Can you work these out from the model? Positions are in its coordinate system, mm. A direction names the side the tool comes from. Round coordinates to 2 decimals unless told otherwise and drop trailing zeros. Loops run counter-clockwise (first coordinate to the right, second up) from the corner with the lowest first, then second, coordinate; pieces in that order, holes last. Notation, with made-up numbers: M -32.75,15 L -23.75,15 A33 ccw -23.75,50 Z; hole C -29,5.5 d6. An arc over 180 degrees is marked long. Return JSON: item names as keys, results as strings.
```python
from build123d import *

# Parameters (mm, degrees)
SKETCH1_W               = 6.3
SKETCH1_H               = 5.3
BOSS_EXTRUDE1_DEPTH     = 2
SKETCH2_W               = 0.25
SKETCH2_H               = 1.2
BOSS_EXTRUDE2_DEPTH     = 1.3
LPATTERN1_COUNT         = 8
LPATTERN1_PITCH         = 0.65
MIRROR1_COPY_1_SKETCH_W = 0.25
MIRROR1_COPY_1_SKETCH_H = 1.2
MIRROR1_COPY_1_DEPTH    = 1.3
MIRROR1_COPY_2_SKETCH_W = 0.25
MIRROR1_COPY_2_SKETCH_H = 1.2
MIRROR1_COPY_2_DEPTH    = 1.3
MIRROR1_COPY_3_SKETCH_W = 0.25
MIRROR1_COPY_3_SKETCH_H = 1.2
MIRROR1_COPY_3_DEPTH    = 1.3
MIRROR1_COPY_4_SKETCH_W = 0.25
MIRROR1_COPY_4_SKETCH_H = 1.2
MIRROR1_COPY_4_DEPTH    = 1.3
MIRROR1_COPY_5_SKETCH_W = 0.25
MIRROR1_COPY_5_SKETCH_H = 1.2
MIRROR1_COPY_5_DEPTH    = 1.3
MIRROR1_COPY_6_SKETCH_W = 0.25
MIRROR1_COPY_6_SKETCH_H = 1.2
MIRROR1_COPY_6_DEPTH    = 1.3
MIRROR1_COPY_7_SKETCH_W = 0.25
MIRROR1_COPY_7_SKETCH_H = 1.2
MIRROR1_COPY_7_DEPTH    = 1.3


with BuildPart() as part:
    # Sketch1 → Boss-Extrude1 (new body)
    with BuildSketch(Plane(origin=(0, 0, 0), x_dir=(1, 0, 0), z_dir=(0, 1, 0))):
        Rectangle(SKETCH1_W, SKETCH1_H)
    extrude(amount=BOSS_EXTRUDE1_DEPTH)

    # Sketch2 → Boss-Extrude2 (add)
    with BuildSketch(Plane.XY.offset(2.65)):
        with Locations((-2.28, 0.6)):
            Rectangle(SKETCH2_W, SKETCH2_H)
    boss_extrude2 = extrude(amount=BOSS_EXTRUDE2_DEPTH)

    # LPattern1: Boss-Extrude2 ×8
    with Locations(*[(i * LPATTERN1_PITCH, 0, 0) for i in range(1, LPATTERN1_COUNT)]):
        add(boss_extrude2)

    # Mirror1: Boss-Extrude2 across plane
    add(boss_extrude2.mirror(Plane.XY))

    # Mirror1 copy 1 sketch → Mirror1 copy 1 (add)
    with BuildSketch(Plane(origin=(0.65, 0, -2.65), x_dir=(1, 0, 0), z_dir=(0, 0, -1))):
        with Locations((-2.28, -0.6)):
            Rectangle(MIRROR1_COPY_1_SKETCH_W, MIRROR1_COPY_1_SKETCH_H)
    extrude(amount=MIRROR1_COPY_1_DEPTH)

    # Mirror1 copy 2 sketch → Mirror1 copy 2 (add)
    with BuildSketch(Plane(origin=(1.3, 0, -2.65), x_dir=(1, 0, 0), z_dir=(0, 0, -1))):
        with Locations((-2.28, -0.6)):
            Rectangle(MIRROR1_COPY_2_SKETCH_W, MIRROR1_COPY_2_SKETCH_H)
    extrude(amount=MIRROR1_COPY_2_DEPTH)

    # Mirror1 copy 3 sketch → Mirror1 copy 3 (add)
    with BuildSketch(Plane(origin=(1.95, 0, -2.65), x_dir=(1, 0, 0), z_dir=(0, 0, -1))):
        with Locations((-2.28, -0.6)):
            Rectangle(MIRROR1_COPY_3_SKETCH_W, MIRROR1_COPY_3_SKETCH_H)
    extrude(amount=MIRROR1_COPY_3_DEPTH)

    # Mirror1 copy 4 sketch → Mirror1 copy 4 (add)
    with BuildSketch(Plane(origin=(2.6, 0, -2.65), x_dir=(1, 0, 0), z_dir=(0, 0, -1))):
        with Locations((-2.28, -0.6)):
            Rectangle(MIRROR1_COPY_4_SKETCH_W, MIRROR1_COPY_4_SKETCH_H)
    extrude(amount=MIRROR1_COPY_4_DEPTH)

    # Mirror1 copy 5 sketch → Mirror1 copy 5 (add)
    with BuildSketch(Plane(origin=(3.25, 0, -2.65), x_dir=(1, 0, 0), z_dir=(0, 0, -1))):
        with Locations((-2.28, -0.6)):
            Rectangle(MIRROR1_COPY_5_SKETCH_W, MIRROR1_COPY_5_SKETCH_H)
    extrude(amount=MIRROR1_COPY_5_DEPTH)

    # Mirror1 copy 6 sketch → Mirror1 copy 6 (add)
    with BuildSketch(Plane(origin=(3.9, 0, -2.65), x_dir=(1, 0, 0), z_dir=(0, 0, -1))):
        with Locations((-2.28, -0.6)):
            Rectangle(MIRROR1_COPY_6_SKETCH_W, MIRROR1_COPY_6_SKETCH_H)
    extrude(amount=MIRROR1_COPY_6_DEPTH)

    # Mirror1 copy 7 sketch → Mirror1 copy 7 (add)
    with BuildSketch(Plane(origin=(4.55, 0, -2.65), x_dir=(1, 0, 0), z_dir=(0, 0, -1))):
        with Locations((-2.28, -0.6)):
            Rectangle(MIRROR1_COPY_7_SKETCH_W, MIRROR1_COPY_7_SKETCH_H)
    extrude(amount=MIRROR1_COPY_7_DEPTH)


solid = part.part
```
Q1. On a 3-axis mill with a long thin cutter (end or side, diameter ignored), from which of +Z, -Z, +X, -X, +Y, -Y can I reach the whole of each face in a straight line? I mean faces 5 (the flat face through (-0.855, 1, -3)), 6 (the flat face through (-0.205, 1, 3)). Say none if no direction works.
Results:
{"face 5": "-Z, +Y, -Y", "face 6": "+Z, +Y, -Y"}
Q2. Suppose I cut it at B-B, the plane x = 1. Please give me the cut outline in (y, z), plus the area to 3 significant figures.
Results:
{"outline": "M 0,-3.95 L 1.2,-3.95 L 1.2,-2.65 L 2,-2.65 L 2,2.65 L 1.2,2.65 L 1.2,3.95 L 0,3.95 Z", "area": "13.7 mm2"}
Q3. Suppose I cut it at C-C, the plane y = 1.6. Please give me the cut outline in (x, z).
Results:
{"outline": "M -3.15,-2.65 L 3.15,-2.65 L 3.15,2.65 L -3.15,2.65 Z"}
Q4. Thinking about a two-plate mould opening in X: for faces 1 (the flat face through (1.095, 1, -3)), 2 (the flat face through (1.495, 1, -3)), 3 (the flat face through (-2.405, 1, 3)), 4 (the flat face through (2.395, 1, 3)), which applies, pulls with the +X half, pulls with the -X half, needs draft (parallel to the pull), parting line crosses it, or undercut?
Results:
{"face 1": "undercut", "face 2": "undercut", "face 3": "pulls with the -X half", "face 4": "pulls with the +X half"}
Q5. Suppose I cut it at A-A, the plane z = -3. State how many separate pieces and enclosed holes the cut face has, plus the area to 3 significant figures.
Results:
{"separate pieces": "8", "enclosed holes": "0", "area": "2.40 mm2"}
Q6. Suppose I cut it at D-D, the plane x = 0. Please give me the cut outline in (y, z), plus the area to 3 significant figures.
Results:
{"outline": "M 0,-2.65 L 2,-2.65 L 2,2.65 L 0,2.65 Z", "area": "10.6 mm2"}
Q7. I'm going to push flat-ended pins straight in: pin 1 Ø0.6 at (y, z) = (1, -3) entering from +X (3 decimals); pin 2 Ø0.6 at (y, z) = (1, -3.5) entering from -X (3 decimals). Where does each tip first touch, or does it pass through?
Results:
{"pin 1": "stops at x = 2.395", "pin 2": "stops at x = -2.405"}
Q8. If I drill on line 1 along Y through (x, z) = (-2.25, 3); line 2 along Z through (x, y) = (0, 0.7), over which ranges is the centre line in solid material (lowest first)?
Results:
{"line 1": "y = 0 to 1.2", "line 2": "z = -2.65 to 2.65"}
